from build123d import *

# Parameters (mm, degrees)
SKETCH_1_R          = 12.5
EXTRUDE_1_DEPTH     = 15
SKETCH_2_R          = 25
EXTRUDE_2_DEPTH     = 5.6
SKETCH_3_R          = 4.95
CUT_EXTRUDE_1_DEPTH = 39.405728739
CUT_EXTRUDE_2_DEPTH = 39.405728739
SKETCH_5_R          = 1.3
CUT_EXTRUDE_3_DEPTH = 46.552167896
SKETCH_6_R          = 1.6
CUT_EXTRUDE_4_DEPTH = 35.003676367
EXTRUDE_START       = 0.5
SKETCH_7_R          = 13.5
SKETCH_7_R_2        = 12.5
EXTRUDE_3_DEPTH     = 0.5
CUT_EXTRUDE_6_DEPTH = 35.003676367
CUT_EXTRUDE_7_DEPTH = 15
FILLET_3_R          = 5
FILLET_4_R          = 1
CUT_EXTRUDE_START   = -15
SKETCH_11_R         = 1.65
SKETCH_11_R_2       = 1.3
CUT_EXTRUDE_8_DEPTH = 15


with BuildPart() as part:
    # ｽｹｯﾁ1 → ﾎﾞｽ - 押し出し1 (new body)
    with BuildSketch(Plane(origin=(0, 0, 0), x_dir=(0, 0, -1), z_dir=(1, 0, 0))):
        Circle(SKETCH_1_R)
    extrude(amount=EXTRUDE_1_DEPTH)

    # ｽｹｯﾁ2 → ﾎﾞｽ - 押し出し2 (add)
    with BuildSketch(Plane(origin=(15, 0, 0), x_dir=(0, 0, -1), z_dir=(1, 0, 0))):
        Circle(SKETCH_2_R)
    extrude(amount=-EXTRUDE_2_DEPTH)

    # ｽｹｯﾁ3 → ｶｯﾄ - 押し出し1 (cut, through all)
    with BuildSketch(Plane(origin=(15, 0, 0), x_dir=(0, 0, -1), z_dir=(1, 0, 0))):
        Circle(SKETCH_3_R)
    extrude(amount=-CUT_EXTRUDE_1_DEPTH, mode=Mode.SUBTRACT)

    # ｽｹｯﾁ4 → ｶｯﾄ - 押し出し2 (cut, through all)
    with BuildSketch(Plane(origin=(15, 0, 0), x_dir=(0, 0, -1), z_dir=(1, 0, 0))):
        with BuildLine():
            Line((-17.853571071, 17.5), (17.853571071, 17.5))
            ThreePointArc((17.853571071, 17.5), (0, 25), (-17.853571071, 17.5))
        make_face()
        with BuildLine():
            Line((17.853571071, -17.5), (-17.853571071, -17.5))
            ThreePointArc((-17.853571071, -17.5), (0, -25), (17.853571071, -17.5))
        make_face()
    extrude(amount=-CUT_EXTRUDE_2_DEPTH, mode=Mode.SUBTRACT)

    # ｽｹｯﾁ5 → ｶｯﾄ - 押し出し3 (cut, through all)
    with BuildSketch(Plane(origin=(0, 17.5, 0), x_dir=(1, 0, 0), z_dir=(0, 1, 0))):
        with Locations(Location((12.2, 0, 0), (0, 0, 270))):
            Circle(SKETCH_5_R)
    extrude(amount=-CUT_EXTRUDE_3_DEPTH, mode=Mode.SUBTRACT)

    # ｽｹｯﾁ6 → ｶｯﾄ - 押し出し4 (cut, through all)
    with BuildSketch(Plane(origin=(15, 0, 0), x_dir=(0, 0, -1), z_dir=(1, 0, 0))):
        with Locations((-19.05, 0)):
            Circle(SKETCH_6_R)
        with Locations((19.05, 0)):
            Circle(SKETCH_6_R)
    extrude(amount=-CUT_EXTRUDE_4_DEPTH, mode=Mode.SUBTRACT)

    # ｽｹｯﾁ7 → ﾎﾞｽ - 押し出し3 (add)
    with BuildSketch(Plane.ZY.offset(-9.4).offset(EXTRUDE_START)):
        with Locations(Location((0, 0, 0), (0, 0, 180))):
            Circle(SKETCH_7_R)
        Circle(SKETCH_7_R_2, mode=Mode.SUBTRACT)
    extrude(amount=-EXTRUDE_3_DEPTH)

    # ｽｹｯﾁ9 → ｶｯﾄ - 押し出し6 (cut, through all)
    with BuildSketch(Plane(origin=(15, 0, 0), x_dir=(0, 0, -1), z_dir=(1, 0, 0))):
        with BuildLine():
            Line((-17.853571071, -17.5), (-7.5, -17.5))
            Line((-7.5, -17.5), (-22.445895783, -3.669862645))
            ThreePointArc((-22.445895783, -3.669862645), (-24.05, 0), (-22.445895783, 3.669862645))
            Line((-22.445895783, 3.669862645), (-7.5, 17.5))
            Line((-7.5, 17.5), (-17.853571071, 17.5))
            ThreePointArc((-17.853571071, 17.5), (-25, 0), (-17.853571071, -17.5))
        make_face()
        with BuildLine():
            Line((22.445895783, -3.669862645), (7.5, -17.5))
            Line((7.5, -17.5), (17.853571071, -17.5))
            ThreePointArc((17.853571071, -17.5), (25, 0), (17.853571071, 17.5))
            Line((17.853571071, 17.5), (7.5, 17.5))
            Line((7.5, 17.5), (22.445895783, 3.669862645))
            ThreePointArc((22.445895783, 3.669862645), (23.631456041, 2.002563493), (24.05, 0))
            ThreePointArc((24.05, 0), (23.631456041, -2.002563493), (22.445895783, -3.669862645))
        make_face()
    extrude(amount=-CUT_EXTRUDE_6_DEPTH, mode=Mode.SUBTRACT)

    # ｽｹｯﾁ10 → ｶｯﾄ - 押し出し7 (cut)
    with BuildSketch(Plane(origin=(15, 0, 0), x_dir=(0, 0, -1), z_dir=(1, 0, 0))):
        with BuildLine():
            Line((-3.025, 4), (3.025, 4))
            Line((3.025, 4), (3.025, 8.1))
            ThreePointArc((3.025, 8.1), (0, 11.125), (-3.025, 8.1))
            Line((-3.025, 8.1), (-3.025, 4))
        make_face()
    extrude(amount=-CUT_EXTRUDE_7_DEPTH, mode=Mode.SUBTRACT)

    # ﾌｨﾚｯﾄ3
    fillet_3_edges = [part.edges().sort_by_distance(p)[0] for p in [
        (12.2, 17.5, -7.5),
        (12.2, 17.5, 7.5),
        (12.2, -17.5, -7.5),
        (12.2, -17.5, 7.5),
    ]]
    fillet(fillet_3_edges, radius=FILLET_3_R)

    # ﾌｨﾚｯﾄ4
    # the kernel refuses this fillet: 1 mm, written as the material it takes off along each edge
    with BuildSketch(Plane(origin=(-1.021064618, 4, -2.915904662), x_dir=(0, 0, -1), z_dir=(1, 0, 0))) as fillet_4_piece_1:
        with BuildLine():
            CenterArc((0.973519116, 0.502763893), FILLET_4_R, 210.183026769, 18.996983583)
            ThreePointArc((0.319834447, -0.254003148), (0.162538073, -0.123701466), (0, 0))
            Line((0, 0), (0.109095338, 0))
        make_face()
    extrude(amount=17.042129236, mode=Mode.SUBTRACT)
    with BuildSketch(Plane(origin=(-1.021064618, 4, 2.915904662), x_dir=(0, -0.6219076232643732, 0.783090612972508), z_dir=(1, 0, 0))) as fillet_4_piece_2:
        with BuildLine():
            CenterArc((0.449680983, -0.999148644), FILLET_4_R, 92.364416205, 18.996983583)
            Line((0.085431535, -0.067847222), (0, 0))
            ThreePointArc((0, 0), (0.204212924, -0.00421421), (0.408425847, 0))
        make_face()
    extrude(amount=17.042129236, mode=Mode.SUBTRACT)

    # ｽｹｯﾁ11 → ｶｯﾄ - 押し出し8 (cut)
    with BuildSketch(Plane.XZ.offset(17.5).offset(CUT_EXTRUDE_START)):
        with Locations(Location((12.2, 0, 0), (0, 0, 270))):
            Circle(SKETCH_11_R)
        with Locations(Location((12.2, 0, 0), (0, 0, 90))):
            Circle(SKETCH_11_R_2, mode=Mode.SUBTRACT)
    extrude(amount=CUT_EXTRUDE_8_DEPTH, mode=Mode.SUBTRACT)


solid = part.part
Could you check a few things on this model? Use its own coordinates, in mm. A direction names the side the tool comes from. Coordinates: 2 decimals unless noted, no trailing zeros. Order: outer loops, then holes, each group sorted by start corner. A loop starts at its lowest first (then second) coordinate and runs counter-clockwise, first axis right, second up.
Q1. Thinking about a two-plate mould opening in Z: for faces 1 (the cylindrical face through (12.161, 17.165, 7.341)), 2 (the cylindrical face through (7.605, 11.124, -0.067)), 3 (the flat face through (8, 6, 3.025)), 4 (the flat face through (9.4, 10.5, 9)), which applies, released by +Z, released by -Z, zero draft, split by the parting line, or undercut?
Q2. Suppose I cut it at A-A on z = 0. Please give me the cut outline in (x, y) (3 decimals), and give its area (3 significant figures).
Q3. Will these pins go through, and if not, where does the flat tip stop? pin 1 (5 mm diameter, centred on x = 4, z = 7, fed in from -Y); pin 2 (2 mm diameter, centred on x = 10.5, y = 7.5, fed in from +Z); pin 3 (1 mm diameter, centred on y = 9.5, z = -11.5, fed in from -X).
Q4. Suppose I cut it at B-B on x = 12.2. Please give me the cut outline in (y, z) (3 decimals), and give its area (3 significant figures).
Q5. Which directions (+Z, -Z, +X, -X, +Y, -Y) give clear straight access to the entire face, cutting with the end or side of a thin tool? Please do faces 5 (the cylindrical face through (12.239, 0.481, 17.524)), 6 (the cylindrical face through (9.15, 13.18, 2.93)), 7 (the cylindrical face through (13.315, -10.994, 1.216)).
Q6. Suppose I cut it at C-C on x = 10. Please give me the cut outline in (y, z) (3 decimals).
Q7. Please list where these lines run through material, in increasing order: L1, parallel to X at y = -14.5, z = 0; L2, parallel to X at y = 13.25, z = 0; L3, parallel to X at y = 3.5, z = 19.5.
Q8. Suppose I cut it at D-D on y = -8.5. Please give me the cut outline in (x, z), and give its area (3 significant figures).
Answer:
1. face 1: released by +Z
1. face 2: undercut
1. face 3: undercut
1. face 4: zero draft
2. outline: (0, -12.5) - (8.9, -12.5) - (8.9, -13.5) - (9.4, -13.5) - (9.4, -17.5) - (10.55, -17.5) - (10.55, -4.95) - (0, -4.95) - close; (0, 11.125) - (10.9, 11.125) - (10.9, 17.5) - (9.4, 17.5) - (9.4, 13.5) - (8.9, 13.5) - (8.9, 12.5) - (0, 12.5) - close; (13.5, 11.125) - (15, 11.125) - (15, 17.5) - (13.5, 17.5) - close; (13.85, -17.5) - (15, -17.5) - (15, -4.95) - (13.85, -4.95) - close
2. area: 133 mm2
3. pin 1: stops at y = -11.66
3. pin 2: stops at z = 19.39
3. pin 3: stops at x = 9.4
4. outline: (-17.5, -5.542) arc R5 ccw to (-16.17, -8.937) - (-3.67, -22.446) arc R5 ccw to (3.67, -22.446) - (16.17, -8.937) arc R5 ccw to (17.5, -5.542) - (17.5, -1.3) - (10.831, -1.3) arc R3.025 cw to (8.1, -3.025) - (4, -3.025) arc R1 ccw to (3.746, -3.236) arc R4.95 cw to (-4.667, -1.65) - (-17.5, -1.65) - close; (-17.5, 1.65) - (-4.667, 1.65) arc R4.95 cw to (3.746, 3.236) arc R1 ccw to (4, 3.025) - (8.1, 3.025) arc R3.025 cw to (10.831, 1.3) - (17.5, 1.3) - (17.5, 5.542) arc R5 ccw to (16.17, 8.937) - (3.67, 22.446) arc R5 ccw to (-3.67, 22.446) - (-16.17, 8.937) arc R5 ccw to (-17.5, 5.542) - close; hole circle Ø3.2 at (0, -19.05); hole circle Ø3.2 at (0, 19.05)
4. area: 985 mm2
5. face 5: +X, -X
5. face 6: -X
5. face 7: -Y
6. outline: (-17.5, -5.542) arc R5 ccw to (-16.17, -8.937) - (-3.67, -22.446) arc R5 ccw to (3.67, -22.446) - (16.17, -8.937) arc R5 ccw to (17.5, -5.542) - (17.5, 5.542) arc R5 ccw to (16.17, 8.937) - (3.67, 22.446) arc R5 ccw to (-3.67, 22.446) - (-16.17, 8.937) arc R5 ccw to (-17.5, 5.542) - close; hole circle Ø3.2 at (0, -19.05); hole circle Ø3.2 at (0, 19.05); hole (3.746, -3.236) arc R1 cw to (4, -3.025) - (8.1, -3.025) arc R3.025 ccw to (8.1, 3.025) - (4, 3.025) arc R1 cw to (3.746, 3.236) arc R4.95 ccw (long way) to start
7. L1: x = 9.4 to 10.55, 13.85 to 15
7. L2: x = 8.9 to 10.9, 13.5 to 15
7. L3: x = 9.4 to 15
8. outline: (0, -9.17) - (8.9, -9.17) - (8.9, -10.49) - (9.4, -10.49) - (9.4, -17.23) - (15, -17.23) - (15, 17.23) - (9.4, 17.23) - (9.4, 10.49) - (8.9, 10.49) - (8.9, 9.17) - (0, 9.17) - close; hole circle Ø3.3 at (12.2, 0)
8. area: 358 mm2
